Verification items for the finished model (mm, model axes). A direction names the side the tool comes from. Round coordinates to 2 decimals unless told otherwise and drop trailing zeros. Write each loop counter-clockwise with the first axis right and the second up, starting at its lowest first coordinate (ties: lowest second). Pieces come first, ordered by that corner, then holes. Notation, with made-up numbers: (27, 88.25) -> (84, 88.25) arc R23 ccw to (84, 111.25) -> close; hole circle Ø1 at (-31, 48). An arc over 180 degrees is marked (long way). Answer as a JSON object with one key per item and string values. Group by question number.
(1) Sectioned sample at D-D on y = 9. Record the cut outline in (x, z), and give its area (3 significant figures).
(2) Scan lines: L1, parallel to X at y = 8.05, z = 0; L2, parallel to X at y = 1.75, z = 5.25; L3, parallel to Z at x = -16, y = 3.5. Record each from-to range of solid material in increasing order. Write a range as from..to.
(3) Draft check along X on faces 4 (the face through (-14, 3, 7.848)), 5 (the face through (-5.393, 3.451, -3.159)), 6 (the face through (10.31, 9.4, -0.08)). Enter one of: released by +X, released by -X, zero draft, split by the parting line, or undercut.
(4) Set-up check for faces 1 (the face through (5.393, 3.451, 3.159)), 2 (the face through (-23.338, 3, 1)), 3 (the face through (-21, 5.396, 0)): record each of +Z, -Z, +X, -X, +Y, -Y from which the full face is reachable in a straight line by a thin tool's end or side.
(5) Sectioned sample at B-B on x = -17.5. Record the cut outline in (y, z).
(6) Gauge pin test, flat ends, axial feed: pin 1 Ø0.7 at (y, z) = (7.5, 1.5) entering from -X; pin 2 Ø1.5 at (y, z) = (6.5, 3.5) entering from -X; pin 3 Ø5.5 at (x, z) = (0, 0) entering from -Y. Record the tip position at first contact, or that the pin passes through.
(7) Sectioned sample at C-C on z = -2.5. Record the cut outline in (x, y), and give its area (3 significant figures).
(8) Sectioned sample at A-A on y = 2.5. Record the cut outline in (x, z), and give its area (3 significant figures).
```python
from build123d import *

# Parameters (mm, degrees)
SKETCH1_W           = 46.934067204
SKETCH1_H           = 15.695815502
BOSS_EXTRUDE1_DEPTH = 7
SKETCH2_W           = 46.934067204
SKETCH2_H           = 15.695815502
BOSS_EXTRUDE2_DEPTH = 3
SKETCH3_W           = 32.738111576
SKETCH3_H           = 6.605539494
CUT_EXTRUDE1_DEPTH  = 41.57096825
SKETCH4_W           = 9.10377614
SKETCH4_H           = 13.037427907
SKETCH4_W_2         = 10.726428155
CUT_EXTRUDE2_DEPTH  = 10
FILLET1_R           = 2
SKETCH5_R           = 1.732622303
CUT_EXTRUDE3_DEPTH  = 10


with BuildPart() as part:
    # Sketch1 → Boss-Extrude1 (new body)
    with BuildSketch(Plane(origin=(0, 0, 0), x_dir=(1, 0, 0), z_dir=(0, 1, 0))):
        with Locations((-12.583553639, 0)):
            Rectangle(SKETCH1_W, SKETCH1_H)
        Polygon((3.620053236, -6.243280219), (7.216865891, 0.013417956), (3.596812655, 6.256698176), (-3.620053236, 6.243280219), (-7.216865891, -0.013417956), (-3.596812655, -6.256698176), align=None, mode=Mode.SUBTRACT)
    extrude(amount=BOSS_EXTRUDE1_DEPTH)

    # Sketch2 → Boss-Extrude2 (add)
    with BuildSketch(Plane(origin=(0, 7, 0), x_dir=(1, 0, 0), z_dir=(0, 1, 0))):
        with Locations((-12.583553639, 0)):
            Rectangle(SKETCH2_W, SKETCH2_H)
    extrude(amount=BOSS_EXTRUDE2_DEPTH)

    # Sketch3 → Cut-Extrude1 (cut, through all)
    with BuildSketch(Plane.XY.offset(7.847907751)):
        with Locations((-25.336793279, 8.698923123)):
            Rectangle(SKETCH3_W, SKETCH3_H)
    extrude(amount=-CUT_EXTRUDE1_DEPTH, mode=Mode.SUBTRACT)

    # Sketch4 → Cut-Extrude2 (cut)
    with BuildSketch(Plane(origin=(0, 5.396153376, 0), x_dir=(1, 0, 0), z_dir=(0, 1, 0))):
        with Locations((-16.116840413, 0.270231687)):
            Rectangle(SKETCH4_W, SKETCH4_H)
        with Locations((-28.701467889, 0.270231687)):
            Rectangle(SKETCH4_W_2, SKETCH4_H)
    extrude(amount=-CUT_EXTRUDE2_DEPTH, mode=Mode.SUBTRACT)

    # Fillet1
    fillet1_edges = [part.edges().sort_by_distance(p)[0] for p in [
        (0.957871236, 10, -7.847907751),
        (10.883479963, 10, 0),
        (0.957871236, 10, 7.847907751),
        (-8.967737491, 10, 0),
        (10.883479963, 0, 0),
        (-8.967737491, 5.396153376, 0),
        (10.883479963, 5, 7.847907751),
        (10.883479963, 5, -7.847907751),
        (-20.668728483, 2.698076688, 6.248482266),
        (-20.668728483, 2.698076688, -6.788945641),
        (-11.564952343, 2.698076688, -6.788945641),
        (-11.564952343, 2.698076688, 6.248482266),
        (-23.338253811, 2.698076688, -6.788945641),
        (-34.064681966, 2.698076688, 6.248482266),
        (-34.064681966, 2.698076688, -6.788945641),
    ]]
    fillet(fillet1_edges, radius=FILLET1_R)

    # Sketch5 → Cut-Extrude3 (cut)
    with BuildSketch(Plane(origin=(0, 10, 0), x_dir=(1, 0, 0), z_dir=(0, 1, 0))):
        with Locations(Location((0, 0, 0), (0, 0, 270))):
            Circle(SKETCH5_R)
    extrude(amount=-CUT_EXTRUDE3_DEPTH, mode=Mode.SUBTRACT)


solid = part.part
```
Computed values:
{
 "1": {"outline": "(-8.7, -7.58) -> (8.88, -7.58) arc R1.73 ccw to (10.62, -5.85) -> (10.62, 5.85) arc R1.73 ccw to (8.88, 7.58) -> (-8.7, 7.58) -> close; hole circle Ø3.47 at (0, 0)", "area": "282 mm2"},
 "2": {"L1": "-8.97..-1.73, 1.73..10.88", "L2": "-36.05..-33.8, -23.34..-20.4, -11.83..-4.18, 4.19..10.87", "L3": "-7.85..-6.79, 6.25..7.85"},
 "3": {"face 4": "zero draft", "face 5": "undercut", "face 6": "released by +X"},
 "4": {"face 1": "-Y", "face 2": "+Y, -Y", "face 3": "+Z, -Z, -X, +Y"},
 "5": {"outline": "(0, -7.85) -> (5.4, -7.85) -> (5.4, -6.79) -> (0, -6.79) -> close; (0, 6.25) -> (5.4, 6.25) -> (5.4, 7.85) -> (0, 7.85) -> close"},
 "6": {"pin 1": "x = -8.98", "pin 2": "x = -9.83", "pin 3": "y = 7"},
 "7": {"outline": "(-36.05, 0) -> (-34.06, 0) -> (-34.06, 5.4) -> (-36.05, 5.4) -> close; (-23.34, 0) -> (-20.67, 0) -> (-20.67, 5.4) -> (-23.34, 5.4) -> close; (-11.56, 0) -> (-5.77, 0) -> (-5.77, 7) -> (5.78, 7) -> (5.78, 0) -> (8.88, 0) arc R2 ccw to (10.88, 2) -> (10.88, 8) arc R2 ccw to (8.88, 10) -> (-6.97, 10) arc R2 ccw to (-8.97, 8) -> (-8.97, 7.4) arc R2 cw to (-10.97, 5.4) -> (-11.56, 5.4) -> close", "area": "155 mm2"},
 "8": {"outline": "(-36.05, -7.85) -> (8.88, -7.85) arc R2 ccw to (10.88, -5.85) -> (10.88, 5.85) arc R2 ccw to (8.88, 7.85) -> (-36.05, 7.85) -> close; hole (-34.06, -4.79) arc R2 ccw to (-32.06, -6.79) -> (-25.34, -6.79) arc R2 ccw to (-23.34, -4.79) -> (-23.34, 6.25) -> (-32.06, 6.25) arc R2 ccw to (-34.06, 4.25) -> close; hole (-20.67, -4.79) arc R2 ccw to (-18.67, -6.79) -> (-13.56, -6.79) arc R2 ccw to (-11.56, -4.79) -> (-11.56, 4.25) arc R2 ccw to (-13.56, 6.25) -> (-18.67, 6.25) arc R2 ccw to (-20.67, 4.25) -> close; hole (-7.22, 0.01) -> (-3.62, -6.24) -> (3.6, -6.26) -> (7.22, -0.01) -> (3.62, 6.24) -> (-3.6, 6.26) -> close", "area": "347 mm2"}
}
